Answer from the drawing. Dimensions are ordinates in mm from the lowest x, y and z of the part. A direction names the side the tool comes from. Coordinates: 2 decimals unless noted, no trailing zeros. Write each loop counter-clockwise with the first axis right and the second up, starting at its lowest first coordinate (ties: lowest second). Pieces come first, ordered by that corner, then holes.
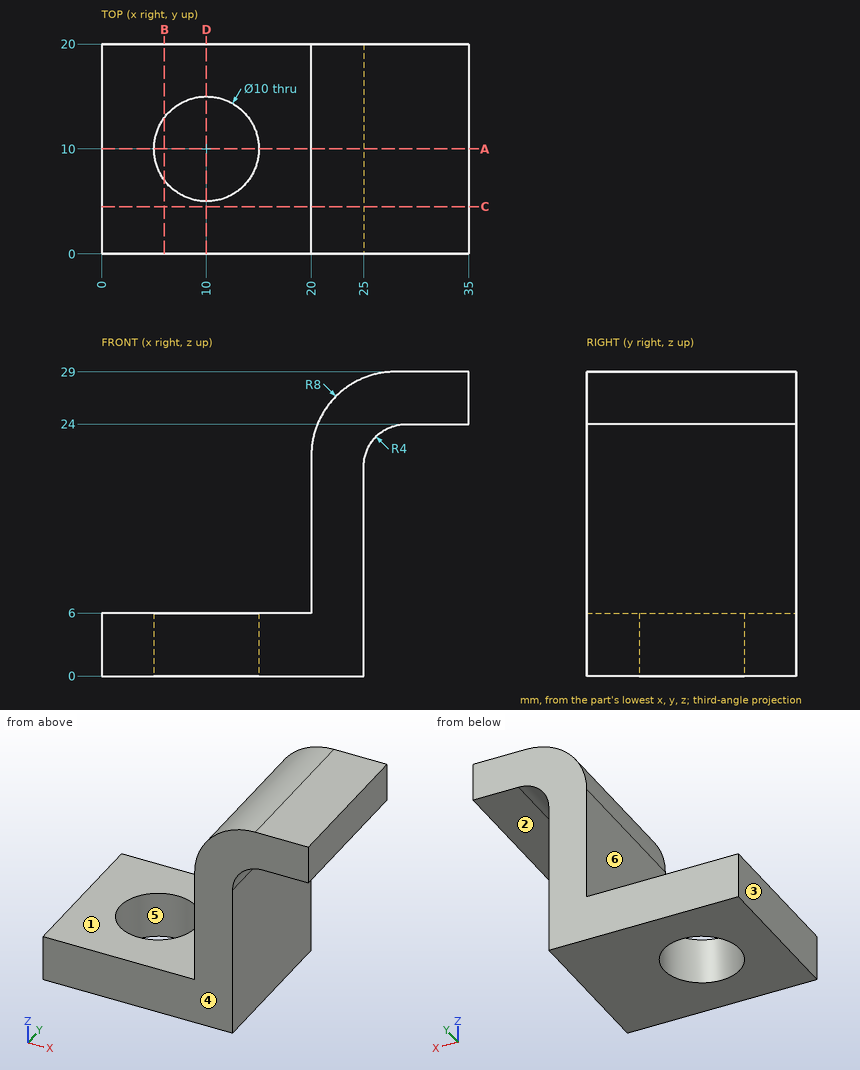
(1) Section D-D, the plane x = 10 is taken. Write down the section's boundary in (y, z), plus the area to 3 significant figures.
(2) Section C-C, the plane y = 4.5 is taken. Write down the section's boundary in (x, z).
(3) Each of these flat-tipped pins is pushed along its axis until it touches: pin 1 (1.5 mm diameter, centred on x = 10, y = 16.5, fed in from +Z); pin 2 (4 mm diameter, centred on y = 15, z = 20.5, fed in from -X); pin 3 (1.5 mm diameter, centred on y = 12, z = 20.5, fed in from +X). Where does it stop, or does it pass through?
(4) Find the intervals of material crossed by probe 1 along Y at (x, z) = (10, 2.9); probe 2 along X at (y, z) = (4, 4); probe 3 along X at (y, z) = (13.75, 9.5), in increasing order.
(5) Section B-B, the plane x = 6 is taken. Write down the section's boundary in (y, z), plus the area to 3 significant figures.
(6) Which of the six approach directions +Z, -Z, +X, -X, +Y, -Y give full straight-line access (tool end or side, diameter ignored) to the marked faces 1, 2 and 3?
(7) Section A-A, the plane y = 10 is taken. Write down the section's boundary in (x, z).
(8) For a pull along Y with two mould halves and no side action, classify the marked faces 4, 5 and 6 as pulls with the +Y half, pulls with the -Y half, needs draft (parallel to the pull), parting line crosses it, or undercut.
Solution:
1. outline: (0, 0) - (5, 0) - (5, 6) - (0, 6) - close; (15, 0) - (20, 0) - (20, 6) - (15, 6) - close
1. area: 60.0 mm2
2. outline: (0, 0) - (25, 0) - (25, 20) arc R4 cw to (29, 24) - (35, 24) - (35, 29) - (28, 29) arc R8 ccw to (20, 21) - (20, 6) - (0, 6) - close
3. pin 1: stops at z = 6
3. pin 2: stops at x = 20
3. pin 3: stops at x = 25.2
4. probe 1: y = 0 to 5, 15 to 20
4. probe 2: x = 0 to 25
4. probe 3: x = 20 to 25
5. outline: (0, 0) - (7, 0) - (7, 6) - (0, 6) - close; (13, 0) - (20, 0) - (20, 6) - (13, 6) - close
5. area: 84.0 mm2
6. face 1: +Z, -X, +Y, -Y
6. face 2: -Z, +X, +Y, -Y
6. face 3: +Z, -Z, -X, +Y, -Y
7. outline: (0, 0) - (5, 0) - (5, 6) - (0, 6) - close; (15, 0) - (25, 0) - (25, 20) arc R4 cw to (29, 24) - (35, 24) - (35, 29) - (28, 29) arc R8 ccw to (20, 21) - (20, 6) - (15, 6) - close
8. face 4: pulls with the -Y half
8. face 5: undercut
8. face 6: needs draft
